Work out the finished part from the listing and answer in its coordinate system (mm). Give positions to 0.01 mm unless a question says otherwise; leave off trailing zeros. Order: outer loops, then holes, each group sorted by start corner. A loop starts at its lowest first (then second) coordinate and runs counter-clockwise, first axis right, second up.
Autodesk Inventor part; units mm, degrees
ref_plane "YZ Plane" through (0, 0, 0) normal (1, 0, 0) x (0, 1, 0)
ref_plane "XZ Plane" through (0, 0, 0) normal (0, 1, 0) x (-1, 0, 0)
ref_plane "XY Plane" through (0, 0, 0) normal (0, 0, 1) x (1, 0, 0)
sketch "Sketch1" plane through (0, 0, 0) normal (0, 1, 0) x (-1, 0, 0)
  line L0 (-7, 37.9777) -> (-7, 79.4722)
  spline S0 degree 3 poles (-7, 79.4722) (-7, 80.2679) (-6.8804, 81.313) (-5.8043, 84.1015) (-4.8936, 85.3942) (-3.1709, 87.6073) (-2.4028, 88.4658) (-2.0131, 89.2627) (-1.9647, 89.4035) (-1.9309, 89.6007) (-1.9254, 89.6626) (-1.9254, 89.7249) knots 0 0 0 0 0.238712 0.238712 0.524177 0.524177 0.81278 0.81278 0.88277 0.88277 0.915008 0.915008 0.915008 0.915008
  line L1 (0, 89.7249) -> (-1.9254, 89.7249)
  line L2 (0, 111.4478) -> (0, 89.7249)
  arc A0 (-6.2149, 117.4498) -> (0, 111.4478) centre (-2.5273, 115.0495) ccw
  line L3 (-135.9053, 117.4498) -> (-6.2149, 117.4498)
  arc A1 (-141.8339, 111.5213) -> (-135.9053, 117.4498) centre (-139.8146, 115.4305) ccw
  line L4 (-141.8339, 89.7249) -> (-141.8339, 111.5213)
  line L5 (-139.9085, 89.7249) -> (-141.8339, 89.7249)
  spline S1 degree 3 poles (-134.8339, 79.4722) (-134.8339, 80.1182) (-134.9165, 80.7597) (-135.2383, 82.0916) (-135.4922, 82.7684) (-136.3337, 84.5039) (-137.0038, 85.4638) (-138.2583, 87.0963) (-138.8405, 87.7821) (-139.5233, 88.7046) (-139.7055, 88.9932) (-139.8538, 89.363) (-139.888, 89.4816) (-139.9062, 89.645) (-139.9085, 89.685) (-139.9085, 89.7249) knots -1.843204 -1.843204 -1.843204 -1.843204 -1.717345 -1.717345 -1.576636 -1.576636 -1.342905 -1.342905 -1.132569 -1.132569 -0.995579 -0.995579 -0.934295 -0.934295 -0.914246 -0.914246 -0.914246 -0.914246
  line L6 (-134.8339, 79.4722) -> (-134.8339, 37.9777)
  spline S2 degree 3 poles (-134.8339, 37.9777) (-134.8339, 37.182) (-134.9535, 36.1368) (-136.0296, 33.3484) (-136.9403, 32.0557) (-138.663, 29.8425) (-139.4311, 28.984) (-139.8208, 28.1872) (-139.8692, 28.0464) (-139.903, 27.8492) (-139.9085, 27.7873) (-139.9085, 27.7249) knots 0 0 0 0 0.238712 0.238712 0.524177 0.524177 0.81278 0.81278 0.88277 0.88277 0.915008 0.915008 0.915008 0.915008
  line L7 (-141.8339, 27.7249) -> (-139.9085, 27.7249)
  line L8 (-141.8339, 5.9286) -> (-141.8339, 27.7249)
  arc A2 (-135.9053, 0) -> (-141.8339, 5.9286) centre (-139.8146, 2.0193) ccw
  line L9 (-6.0879, 0) -> (-135.9053, 0)
  arc A3 (0, 6.0879) -> (-6.0879, 0) centre (-2.4003, 2.4003) ccw
  line L10 (0, 27.7249) -> (0, 6.0879)
  line L11 (-1.9254, 27.7249) -> (0, 27.7249)
  spline S3 degree 3 poles (-7, 37.9777) (-7, 37.3317) (-6.9174, 36.6902) (-6.5955, 35.3583) (-6.3417, 34.6814) (-5.5001, 32.9459) (-4.8301, 31.986) (-3.5755, 30.3535) (-2.9934, 29.6677) (-2.3106, 28.7453) (-2.1284, 28.4567) (-1.9801, 28.0868) (-1.9459, 27.9682) (-1.9277, 27.8049) (-1.9254, 27.7649) (-1.9254, 27.7249) knots -1.843204 -1.843204 -1.843204 -1.843204 -1.717345 -1.717345 -1.576636 -1.576636 -1.342905 -1.342905 -1.132569 -1.132569 -0.995579 -0.995579 -0.934295 -0.934295 -0.914246 -0.914246 -0.914246 -0.914246
  circle A4 centre (-121.8339, 20) radius 2.75
  line L12 (-121.8339, 24.7343) -> (-117.7339, 22.3671)
  line L13 (-117.7339, 22.3671) -> (-117.7339, 17.6329)
  line L14 (-117.7339, 17.6329) -> (-121.8339, 15.2657)
  line L15 (-121.8339, 15.2657) -> (-125.9339, 17.6329)
  line L16 (-125.9339, 17.6329) -> (-125.9339, 22.3671)
  line L17 (-125.9339, 22.3671) -> (-121.8339, 24.7343)
  line L18 (-134.8339, 39.0386) -> (-134.8339, 78.4112)
  line L19 (-134.8339, 58.7249) -> (-125.9339, 58.7249)
  line L20 (-70.9966, 0) -> (-70.9966, 6.0879)
  line L21 (-117.7339, 95.0827) -> (-117.7339, 99.817)
  line L22 (-117.7339, 99.817) -> (-121.8339, 102.1841)
  line L23 (-125.9339, 95.0827) -> (-121.8339, 92.7156)
  line L24 (-125.9339, 99.817) -> (-125.9339, 95.0827)
  circle A5 centre (-121.8339, 97.4498) radius 2.75
  line L25 (-121.8339, 102.1841) -> (-125.9339, 99.817)
  line L26 (-121.8339, 92.7156) -> (-117.7339, 95.0827)
  line L27 (-24.2593, 22.3671) -> (-24.2593, 17.6329)
  line L28 (-20.1593, 24.7343) -> (-24.2593, 22.3671)
  line L29 (-24.2593, 17.6329) -> (-20.1593, 15.2657)
  circle A6 centre (-20.1593, 20) radius 2.75
  line L30 (-16.0593, 17.6329) -> (-16.0593, 22.3671)
  line L31 (-20.1593, 15.2657) -> (-16.0593, 17.6329)
  line L32 (-16.0593, 22.3671) -> (-20.1593, 24.7343)
  line L33 (-20.1593, 92.7156) -> (-24.2593, 95.0827)
  line L34 (-24.2593, 95.0827) -> (-24.2593, 99.817)
  line L35 (-16.0593, 99.817) -> (-16.0593, 95.0827)
  circle A7 centre (-20.1593, 97.4498) radius 2.75
  line L36 (-24.2593, 99.817) -> (-20.1593, 102.1841)
  line L37 (-20.1593, 102.1841) -> (-16.0593, 99.817)
  line L38 (-16.0593, 95.0827) -> (-20.1593, 92.7156)
  circle A8 centre (-121.8339, 20) radius 7.5
  circle A9 centre (-121.8339, 97.4498) radius 7.5
  circle A10 centre (-20.1593, 20) radius 7.5
  circle A11 centre (-20.1593, 97.4498) radius 7.5
  line L39 (26.5034, 108.7249) -> (-168.4966, 108.7249) construction
  line L40 (26.5034, 118.7249) -> (-168.4966, 118.7249)
  line L41 (-168.4966, 98.7249) -> (26.5034, 98.7249)
  arc A12 (26.5034, 98.7249) -> (26.5034, 118.7249) centre (26.5034, 108.7249) ccw
  arc A13 (-168.4966, 118.7249) -> (-168.4966, 98.7249) centre (-168.4966, 108.7249) ccw
  circle A14 centre (26.5034, 108.7249) radius 3.6
  circle A15 centre (-168.4966, 108.7249) radius 3.6
  line L42 (-121.8339, 97.4498) -> (-20.1593, 97.4498)
  line L43 (-20.1593, 97.4498) -> (-20.1593, 20)
  line L44 (26.5034, 8.7249) -> (26.5034, 108.7249)
  line L45 (-168.4966, 108.7249) -> (-168.4966, 8.7249)
  line L46 (26.5034, 8.7249) -> (-168.4966, 8.7249) construction
  line L47 (26.5034, 18.7249) -> (-168.4966, 18.7249)
  line L48 (-168.4966, -1.2751) -> (26.5034, -1.2751)
  arc A16 (26.5034, -1.2751) -> (26.5034, 18.7249) centre (26.5034, 8.7249) ccw
  arc A17 (-168.4966, 18.7249) -> (-168.4966, -1.2751) centre (-168.4966, 8.7249) ccw
  circle A18 centre (26.5034, 8.7249) radius 3.6
  circle A19 centre (-168.4966, 8.7249) radius 3.6
  line L49 (-20.1593, 20) -> (-20.1593, 97.4498) construction
  line L50 (-10.1593, 18.7249) -> (-10.1593, 98.7249)
  line L51 (-30.1593, 98.7249) -> (-30.1593, 18.7249)
  line L52 (-121.8339, 20) -> (-121.8339, 97.4498) construction
  line L53 (-111.8339, 18.7249) -> (-111.8339, 98.7249)
  line L54 (-131.8339, 98.7249) -> (-131.8339, 18.7249)
  point P0 (0, 0)
  point P1 (0, 0)
  point P2 (-16.0593, 58.7249)
  point P3 (-70.9966, 108.7249)
  point P4 (-70.9966, 97.4498)
  point P5 (26.5034, 58.7249)
  point P6 (-20.1593, 58.7249)
  point P7 (-70.9966, 8.7249)
  point P8 (-20.1593, 58.7249)
  point P9 (-121.8339, 58.7249)
  dimension "d0" = 5.5
  dimension "d1" = 8.2
  dimension "d2" = 20
  dimension "d3" = 20
  dimension "d4" = 15
  dimension "d5" = 195
  dimension "d6" = 20
  dimension "d7" = 7.2
  dimension "d8" = 7.2
  dimension "d9" = 100
  dimension "d10" = 20
  dimension "d11" = 7.2
  dimension "d12" = 7.2
extrude "Extrusion1" add sketch "Sketch1" along normal blind 4 contours L47 A16 L48 A17 L8 A2 L9 A3 L10 | L10 A3 L9 A2 L8 L47 A8 A10 | L41 A11 A9 L4 A1 L3 A0 L2 | L2 A0 L3 A1 L4 L41 A13 L40 A12 | L47 A10 L43 A11 L41 L50 | L47 L30 L32 L43 A10 | A10 L47 L27 L29 L31 L30 | L41 L35 L37 L36 L34 A11 | A11 L43 L38 L35 L41 | L47 L51 L42 A11 L43 A10 | A10 L43 L28 L27 L47 | L47 A6 L43 L32 L30 | L30 L31 L29 L27 L47 A6 | L41 L34 L42 A11 | A11 L42 L51 L41 | L41 A7 L34 L36 L37 L35 | L35 L38 L43 A7 L41 | L27 L28 L43 A6 L47 | A11 L42 L34 L33 L43 | L41 A7 L42 L34 | L47 A8 L54 L41 A9 L42 L53 | L33 L34 L42 A7 L43 | L53 L42 A9 L41 | L47 L13 L12 L17 L16 A8 | A8 L47 L16 L15 L14 L13 | L41 L21 L22 L25 L24 A9 | A9 L42 L21 L41 | L47 A4 L16 L17 L12 L13 | L13 L14 L15 L16 L47 A4 | A9 L41 L24 L23 L26 L21 L42 | L41 A5 L24 L25 L22 L21 | L21 L42 A5 L41 | L21 L26 L23 L24 L41 A5 L42
fillet "Fillet1" radius 6 8 edges at (30.1593, 2, 98.7249) (10.1593, 2, 98.7249) (10.1593, 2, 18.7249) (30.1593, 2, 18.7249) (111.8339, 2, 18.7249) (131.8339, 2, 18.7249) (111.8339, 2, 98.7249) (131.8339, 2, 98.7249)
properties part number "Mount Base"
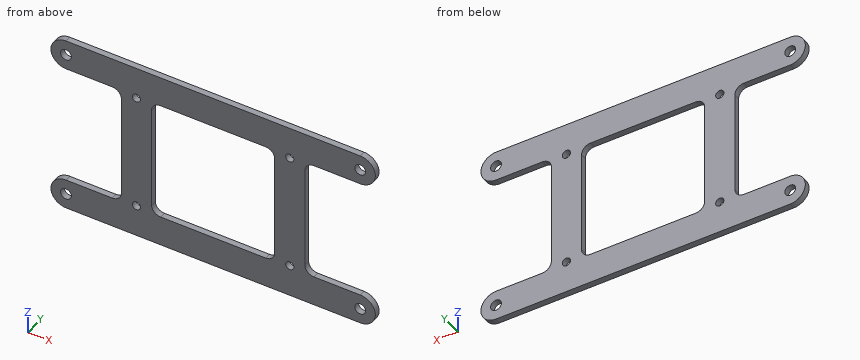
1. The part is cut by section C-C (y = 0.95). State how many separate pieces and enclosed holes the cut face has, then the cut area to 3 significant figures.
Findings below:
separate pieces: 1
enclosed holes: 9
area: 11,400 mm2
2. The part is cut by section A-A (z = 79.5). Write down the section's boundary in (x, y).
Findings below:
outline: (10.16, 0) - (30.16, 0) - (30.16, 4) - (10.16, 4) - close; (111.83, 0) - (131.83, 0) - (131.83, 4) - (111.83, 4) - close
3. Straight lines are drawn through the part: probe 1 along Z at (x, y) = (106, 2.85); probe 2 along X at (y, z) = (3.25, 43); probe 3 along Z at (x, y) = (168.5, 1.85). For each, find the intervals that lie inside material, in ascending order.
Findings below:
probe 1: z = -1.28 to 18.73, 98.72 to 118.72
probe 2: x = 10.16 to 30.16, 111.83 to 131.83
probe 3: z = -1.28 to 5.12, 12.32 to 18.72, 98.72 to 105.12, 112.32 to 118.72
4. Given P1, Ø2, axis at y = 1.5, z = 68.5, coming from the -X side, flat-ended and moving along its own axis, determine where the tip first touches the part or whether it passes through.
Findings below:
P1: stops at x = 10.16
5. The part is cut by section B-B (x = 52). Write down the section's boundary in (y, z), then the cut area to 3 significant figures.
Findings below:
outline: (0, -1.28) - (4, -1.28) - (4, 18.72) - (0, 18.72) - close; (0, 98.72) - (4, 98.72) - (4, 118.72) - (0, 118.72) - close
area: 160 mm2
